For this review, take the finished solid that the model builds, in its own axes (mm). Face numbers are marked on the shaded views. A direction names the side the tool comes from. Round coordinates to 2 decimals unless told otherwise and drop trailing zeros. Loops run counter-clockwise (first coordinate to the right, second up) from the corner with the lowest first, then second, coordinate; pieces in that order, holes last.
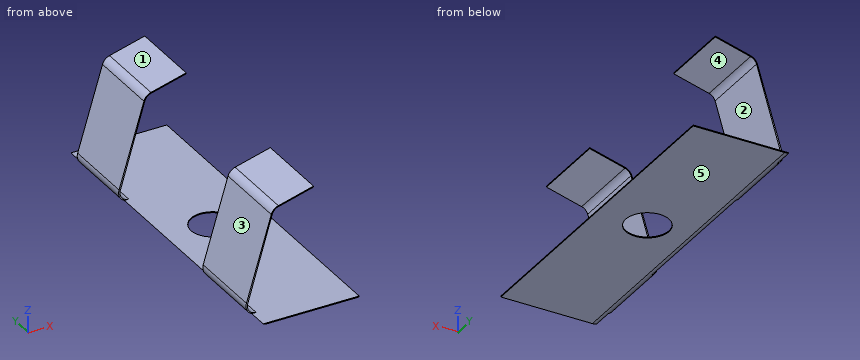
```python
from build123d import *

# Parameters (mm, degrees)
F1_DEPTH = 25.4
F3_W     = 8.148129
F3_H     = 5.55625
F3_W_2   = 7.948229
F3_H_2   = 1.5875
F3_W_3   = 8.837929
F4_DEPTH = 25.4
F5_R     = 1.633227
F6_DEPTH = 25.4


with BuildPart() as f1:
    # F0 (on Front) → F1 (new body)
    with BuildSketch(Plane.XZ):
        with BuildLine():
            Line((-0.561085, 0), (0, 0))
            Line((0, 0), (6.35, 0))
            Line((6.35, 0), (6.35, 0.0762))
            Line((6.35, 0.0762), (-0.561085, 0.0762))
            ThreePointArc((-0.561085, 0.0762), (-1.107829, 0.366771), (-1.172913, 0.982501))
            Line((-1.172913, 0.982501), (0.660235, 7.192055))
            ThreePointArc((0.660235, 7.192055), (0.833247, 7.470557), (1.118945, 7.631408))
            Line((1.118945, 7.631408), (3.776279, 8.343177))
            Line((3.776279, 8.343177), (3.776279, 8.419377))
            Line((3.776279, 8.419377), (1.118945, 7.707608))
            ThreePointArc((1.118945, 7.707608), (0.785934, 7.518885), (0.586698, 7.192055))
            Line((0.586698, 7.192055), (-1.290484, 0.982501))
            ThreePointArc((-1.290484, 0.982501), (-1.172913, 0.307785), (-0.561085, 0))
        make_face()
    extrude(amount=F1_DEPTH)

    # F3 (on offset) → F4 (cut)
    with BuildSketch(Plane.XY.offset(0.0762)):
        with Locations((1.40282, -9.833681)):
            Rectangle(F3_W, F3_H)
        with Locations((0.910564, -0.79375)):
            Rectangle(F3_W_2, F3_H_2)
        with Locations((3.026584, -24.674151)):
            Rectangle(F3_W_3, F3_H_2)
        with Locations((1.40282, -15.389931)):
            Rectangle(F3_W, F3_H)
    extrude(amount=F4_DEPTH, mode=Mode.SUBTRACT)

    # F5 (on face) → F6 (cut)
    with BuildSketch(Plane.XY.offset(0.0762)):
        with Locations((2.596372, -12.611806)):
            Circle(F5_R)
    extrude(amount=-F6_DEPTH, mode=Mode.SUBTRACT)


solid = f1.part
```
(1) Insertion check: pin 1 Ø1.5 at (x, z) = (0.5, 3) entering from +Y; pin 2 Ø1.5 at (x, z) = (0, 6.5) entering from -Y; pin 3 Ø4 at (y, z) = (-3.5, 5.5) entering from -X; pin 4 Ø3.5 at (x, y) = (4.5, -12) entering from +Z. Each pin has a flat end and moves straight along its axis. Give the tip position at first contact, or say it passes through.
(2) Add section B-B (z = 1.25). Give the boundary of the cut face in (x, y).
(3) Add section A-A (x = 3). Give the boundary of the cut face in (y, z).
(4) Add section C-C (y = -22.5). Give the boundary of the cut face in (x, z), plus the area to 3 significant figures.
(5) The part is to be moulded in two halves that separate along Z. For the marked faces 3, 4 and 5, say which applies: pulls with the +Z half, pulls with the -Z half, needs draft (parallel to the pull), parting line crosses it, or undercut.
(6) For the marked faces 1 and 2, list the 3-axis set-ups (+Z, -Z, +X, -X, +Y, -Y) from which the entire face can be reached by the end or side of a thin tool; tool diameter is ignored.
(7) Add section D-D (x = 0). Give the boundary of the cut face in (y, z), plus the area to 3 significant figures.
Outcome:
1. pin 1: passes through
1. pin 2: stops at y = -23.88
1. pin 3: stops at x = -0.53
1. pin 4: stops at z = 0.08
2. outline: (-1.21, -23.88) - (-1.09, -23.88) - (-1.09, -18.17) - (-1.21, -18.17) - close; (-1.21, -7.06) - (-1.09, -7.06) - (-1.09, -1.59) - (-1.21, -1.59) - close
3. outline: (-25.4, 0) - (-14.19, 0) - (-14.19, 0.08) - (-25.4, 0.08) - close; (-23.88, 8.14) - (-18.17, 8.14) - (-18.17, 8.21) - (-23.88, 8.21) - close; (-11.03, 0) - (0, 0) - (0, 0.08) - (-11.03, 0.08) - close; (-7.06, 8.14) - (-1.59, 8.14) - (-1.59, 8.21) - (-7.06, 8.21) - close
4. outline: (-1.29, 0.98) arc R0.76 ccw to (-0.56, 0) - (6.35, 0) - (6.35, 0.08) - (-0.56, 0.08) arc R0.66 cw to (-1.17, 0.98) - (0.66, 7.19) arc R0.66 cw to (1.12, 7.63) - (3.78, 8.34) - (3.78, 8.42) - (1.12, 7.71) arc R0.76 ccw to (0.59, 7.19) - close
4. area: 1.49 mm2
5. face 3: pulls with the +Z half
5. face 4: undercut
5. face 5: pulls with the -Z half
6. face 1: +Z, -X, +Y, -Y
6. face 2: +X, +Y, -Y
7. outline: (-25.4, 0) - (0, 0) - (0, 0.08) - (-25.4, 0.08) - close; (-23.88, 4.96) - (-18.17, 4.96) - (-18.17, 5.25) - (-23.88, 5.25) - close; (-7.06, 4.96) - (-1.59, 4.96) - (-1.59, 5.25) - (-7.06, 5.25) - close
7. area: 5.24 mm2
